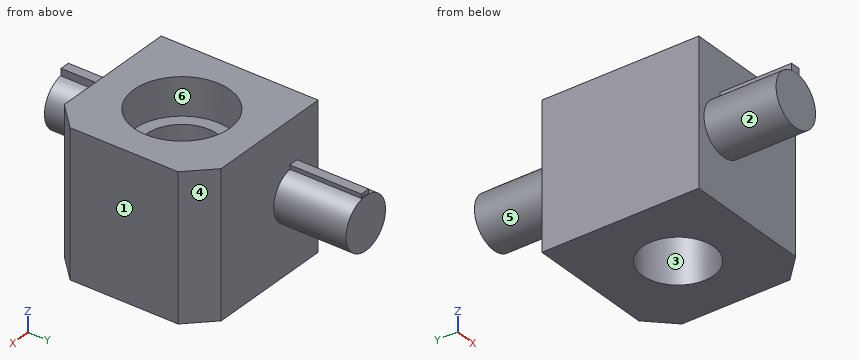
```python
from build123d import *

# Parameters (mm, degrees)
SKETCH2_W           = 6.2
SKETCH2_H           = 6.4
BOSS_EXTRUDE1_DEPTH = 5.86
CHAMFER1_SIZE       = 1
SKETCH5_R           = 1.95
CUT_EXTRUDE3_DEPTH  = 1.52
SKETCH6_R           = 1.45
CUT_EXTRUDE4_DEPTH  = 7.219774916
SKETCH7_R           = 1.06
BOSS_EXTRUDE2_DEPTH = 2.95
SKETCH8_W           = 0.39
SKETCH8_H           = 0.295203358
BOSS_EXTRUDE3_DEPTH = 2.92
SKETCH9_R           = 1.06
BOSS_EXTRUDE4_DEPTH = 2.94
SKETCH11_W          = 0.39
SKETCH11_H          = 0.550473967
BOSS_EXTRUDE5_DEPTH = 2.92


with BuildPart() as part:
    # Sketch2 → Boss-Extrude1 (new body)
    with BuildSketch(Plane.XY):
        Rectangle(SKETCH2_W, SKETCH2_H)
    extrude(amount=BOSS_EXTRUDE1_DEPTH)

    # Chamfer1
    chamfer1_edges = [part.edges().sort_by_distance(p)[0] for p in [
        (3.1, 3.2, 2.93),
        (3.1, -3.2, 2.93),
    ]]
    chamfer(chamfer1_edges, length=CHAMFER1_SIZE)

    # Sketch5 → Cut-Extrude3 (cut)
    with BuildSketch(Plane.XY.offset(5.86)):
        Circle(SKETCH5_R)
    extrude(amount=-CUT_EXTRUDE3_DEPTH, mode=Mode.SUBTRACT)

    # Sketch6 → Cut-Extrude4 (cut, through all)
    with BuildSketch(Plane.XY.offset(4.34)):
        Circle(SKETCH6_R)
    extrude(amount=-CUT_EXTRUDE4_DEPTH, mode=Mode.SUBTRACT)

    # Sketch7 → Boss-Extrude2 (add)
    with BuildSketch(Plane(origin=(0, 3.2, 0), x_dir=(1, 0, 0), z_dir=(0, 1, 0))):
        with Locations(Location((-1.775985432, -2.93, 0), (0, 0, 180))):
            Circle(SKETCH7_R)
    extrude(amount=BOSS_EXTRUDE2_DEPTH)

    # Sketch8 → Boss-Extrude3 (add)
    with BuildSketch(Plane(origin=(0, 3.2, 0), x_dir=(1, 0, 0), z_dir=(0, 1, 0))):
        with Locations((-1.775985432, -3.99)):
            Rectangle(SKETCH8_W, SKETCH8_H)
    extrude(amount=BOSS_EXTRUDE3_DEPTH)

    # Sketch9 → Boss-Extrude4 (add)
    with BuildSketch(Plane.XZ.offset(3.2)):
        with Locations((-1.764050238, 2.930792226)):
            Circle(SKETCH9_R)
    extrude(amount=BOSS_EXTRUDE4_DEPTH)

    # Sketch11 → Boss-Extrude5 (add)
    with BuildSketch(Plane.XZ.offset(3.2)):
        with Locations((-1.764050238, 3.990792225)):
            Rectangle(SKETCH11_W, SKETCH11_H)
    extrude(amount=BOSS_EXTRUDE5_DEPTH)


solid = part.part
```
Work out the finished part from the listing and answer in its coordinate system (mm). Face numbers are marked on the shaded views. A direction names the side the tool comes from. Round coordinates to 2 decimals unless told otherwise and drop trailing zeros. Loops run counter-clockwise (first coordinate to the right, second up) from the corner with the lowest first, then second, coordinate; pieces in that order, holes last. Notation, with made-up numbers: M 33,47 L 71,47 A13 ccw 71,52 Z; hole C 7,30.5 d7. An arc over 180 degrees is marked long. Use CSV: the item, a comma, the result in double quotes.
Q1. A tool of negligible diameter and unlimited length cuts with its end or side. For the marked faces 4, 5 and 6, from which of +Z, -Z, +X, -X, +Y, -Y can it reach the whole face along a straight path? Write none if from no direction.
Determined:
face 4,"+Z, -Z, +X, +Y"
face 5,"+Y"
face 6,"+Z"
Q2. The mould has two halves that part along X. Classify the marked faces 1, 2 and 3: pulls with the +X half, pulls with the -X half, needs draft (parallel to the pull), parting line crosses it, or undercut.
Determined:
face 1,"pulls with the +X half"
face 2,"parting line crosses it"
face 3,"undercut"
Q3. Section A-A, the plane x = 0 is taken. Determine the outline of the cut face in (y, z), then the cut area to 3 significant figures.
Determined:
outline,"M -3.2,0 L -1.45,0 L -1.45,4.34 L -1.95,4.34 L -1.95,5.86 L -3.2,5.86 Z; M 1.45,0 L 3.2,0 L 3.2,5.86 L 1.95,5.86 L 1.95,4.34 L 1.45,4.34 Z"
area,"19.0 mm2"
Q4. Section D-D, the plane x = -2.25 is taken. Determine the outline of the cut face in (y, z), then the cut area to 3 significant figures.
Determined:
outline,"M -6.14,1.99 L -3.2,1.99 L -3.2,0 L 3.2,0 L 3.2,1.98 L 6.15,1.98 L 6.15,3.88 L 3.2,3.88 L 3.2,5.86 L -3.2,5.86 L -3.2,3.87 L -6.14,3.87 Z"
area,"48.6 mm2"
Q5. Section C-C, the plane y = 0.5 is taken. Determine the outline of the cut face in (x, z), then the cut area to 3 significant figures.
Determined:
outline,"M -3.1,0 L -1.36,0 L -1.36,4.34 L -1.88,4.34 L -1.88,5.86 L -3.1,5.86 Z; M 1.36,0 L 3.1,0 L 3.1,5.86 L 1.88,5.86 L 1.88,4.34 L 1.36,4.34 Z"
area,"18.8 mm2"
Q6. Consider L1, parallel to Y at x = 0, z = 1.95; L2, parallel to Y at x = 0, z = 4.7; L3, parallel to X at y = -3.5, z = 4.15. Determine where each line is inside the solid, lowest interval first.
Determined:
L1,"-3.2 to -1.45, 1.45 to 3.2"
L2,"-3.2 to -1.95, 1.95 to 3.2"
L3,"-1.96 to -1.57"
Q7. Each of these flat-tipped pins is pushed along its axis until it touches: pin 1 (2 mm diameter, centred on y = 4, z = 2, fed in from +X); pin 2 (2.5 mm diameter, centred on x = 0, y = 0, fed in from -Z). Where does it stop, or does it pass through?
Determined:
pin 1,"x = 2.3"
pin 2,"through"
Q8. Section B-B, the plane z = 4.9 is taken. Determine the outline of the cut face in (x, y).
Determined:
outline,"M -3.1,-3.2 L 2.1,-3.2 L 3.1,-2.2 L 3.1,2.2 L 2.1,3.2 L -3.1,3.2 Z; hole C 0,0 d3.9"
